Job drawing, mm, ordinate dimensions from the low corner. One solid piece. Round coordinates to 2 decimals unless told otherwise and drop trailing zeros. Loops run counter-clockwise (first coordinate to the right, second up) from the corner with the lowest first, then second, coordinate; pieces in that order, holes last.
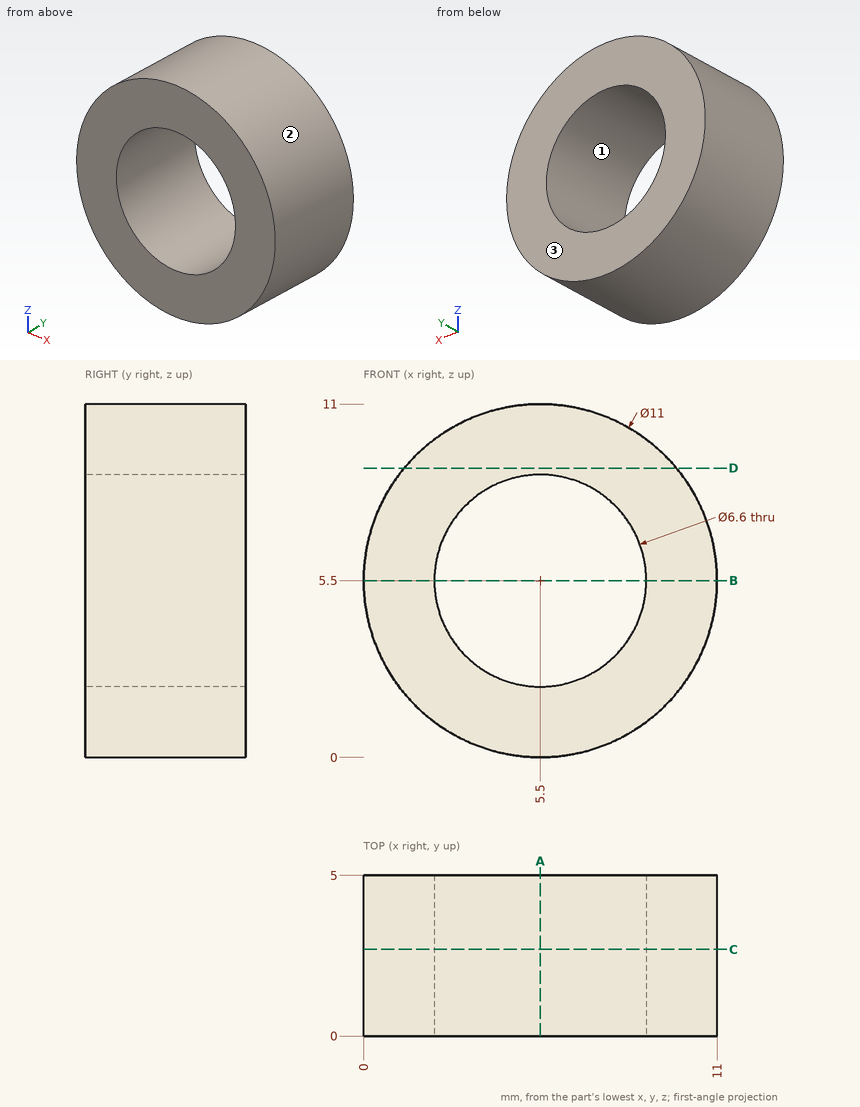
Item 1: Probe line 1 (Z direction, x = 5.5, y = 3.4); line 2 (X direction, y = 3.1, z = 3); line 3 (Z direction, x = 7.5, y = 2.7). List the from-to ranges inside material, lowest first.
Answers follow:
line 1: z = 0 to 2.2, 8.8 to 11
line 2: x = 0.6 to 3.35, 7.65 to 10.4
line 3: z = 0.38 to 2.88, 8.12 to 10.62
Item 2: Cut at D-D, the plane z = 9. Give the cut face in (x, y), plus the area to 3 significant figures.
Answers follow:
outline: (1.26, 0) - (9.74, 0) - (9.74, 5) - (1.26, 5) - close
area: 42.4 mm2
Item 3: Cut at C-C, the plane y = 2.7. Give the cut face in (x, z), plus the area to 3 significant figures.
Answers follow:
outline: circle Ø11 at (5.5, 5.5); hole circle Ø6.6 at (5.5, 5.5)
area: 60.8 mm2
Item 4: Cut at B-B, the plane z = 5.5. Give the cut face in (x, y), plus the area to 3 significant figures.
Answers follow:
outline: (0, 0) - (2.2, 0) - (2.2, 5) - (0, 5) - close; (8.8, 0) - (11, 0) - (11, 5) - (8.8, 5) - close
area: 22.0 mm2
Item 5: Flat gauge pins, fed straight in: P1, Ø3, axis at y = 4.5, z = 7.5, coming from the -X side; P2, Ø1.5, axis at x = 7, y = 1.5, coming from the +Z side; P3, Ø2, axis at x = 8.5, y = 3.5, coming from the -Z side. Where does each tip first touch, or does it go through?
Answers follow:
P1: stops at x = 0.02
P2: stops at z = 10.95
P3: stops at z = 0.38
Item 6: Two-plate mould, pull along X, no slides. Class the marked faces 1, 2 and 3: released by +X, released by -X, zero draft, split by the parting line, or undercut.
Answers follow:
face 1: undercut
face 2: split by the parting line
face 3: zero draft
Item 7: Cut at A-A, the plane x = 5.5. Give the cut face in (y, z).
Answers follow:
outline: (0, 0) - (5, 0) - (5, 2.2) - (0, 2.2) - close; (0, 8.8) - (5, 8.8) - (5, 11) - (0, 11) - close
